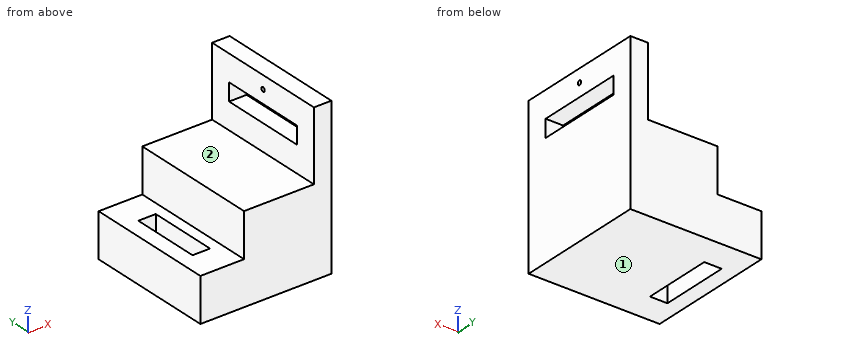
```python
from build123d import *

# Parameters (mm, degrees)
F1_DEPTH = 150
F2_W     = 100
F2_H     = 20
F3_DEPTH = 20.001
F4_R     = 2.5
F5_DEPTH = 20.001
F6_W     = 20
F6_H     = 80
F7_DEPTH = 25.4
F8_W     = 20
F8_H     = 80
F9_DEPTH = 75.401


with BuildPart() as f1:
    # F0 (on Front) → F1 (new body)
    with BuildSketch(Plane.XZ):
        Polygon((75, -90), (75, 90), (55, 90), (55, 10), (-25, 10), (-25, -40), (-75, -40), (-75, -90), align=None)
    extrude(amount=F1_DEPTH)

    # F2 (on face) → F3 (cut, through all)
    with BuildSketch(Plane(origin=(55, 0, 0), x_dir=(0, -1, 0), z_dir=(-1, 0, 0))):
        with Locations((75, 50)):
            Rectangle(F2_W, F2_H)
    extrude(amount=-F3_DEPTH, mode=Mode.SUBTRACT)

    # F4 (on face) → F5 (cut, through all)
    with BuildSketch(Plane(origin=(55, 0, 0), x_dir=(0, -1, 0), z_dir=(-1, 0, 0))):
        with Locations((75, 75)):
            Circle(F4_R)
    extrude(amount=-F5_DEPTH, mode=Mode.SUBTRACT)

    # F6 (on face) → F7 (join)
    with BuildSketch(Plane.XY.offset(-40)):
        with Locations((-47.3200663872, -75.7392449304)):
            Rectangle(F6_W, F6_H)
    extrude(amount=F7_DEPTH)

    # F8 (on face) → F9 (cut, through all)
    with BuildSketch(Plane.XY.offset(-14.6)):
        with Locations((-47.3200663872, -75.7392449304)):
            Rectangle(F8_W, F8_H)
    extrude(amount=-F9_DEPTH, mode=Mode.SUBTRACT)


solid = f1.part
```
For this review, take the finished solid that the model builds, in its own axes (mm). Face numbers are marked on the shaded views. A direction names the side the tool comes from. Coordinates: 2 decimals unless noted, no trailing zeros. Loops run counter-clockwise (first coordinate to the right, second up) from the corner with the lowest first, then second, coordinate; pieces in that order, holes last. Notation, with made-up numbers: (65, -24.5) - (94, -24.5) arc R17 cw to (94, -5.5) - close; hole circle Ø5 at (-31.75, 47.25). An arc over 180 degrees is marked (long way). Use one line per item in the form item = value. Start each with the question number.
1) Take a section at C-C (y = -104). State the section outline as (x, z) points.
2) Take a section at D-D (y = -75). State the section outline as (x, z) points.
3) Take a section at B-B (z = 75). State the section outline as (x, y) points.
4) For pin 1 (8 mm diameter, centred on x = 8, y = -55, fed in from +Z), flat-tipped, find the tip position at first contact; note if it passes through.
5) For the marked faces 1 and 2, list the 3-axis set-ups (+Z, -Z, +X, -X, +Y, -Y) from which the entire face can be reached by the end or side of a thin tool; tool diameter is ignored.
6) Take a section at A-A (x = -46). State the section outline as (y, z) points.
7) To check wall thickness, follow probe 1 along Z at (x, y) = (64, -75); probe 2 along X at (y, z) = (-80, 27); probe 3 along X at (y, z) = (-47, -49). State the ranges of each line that lie inside material, in increasing order. Write a range as from..to.
From the geometry:
q1.outline = (-75, -90) - (-57.32, -90) - (-57.32, -40) - (-75, -40) - close; (-37.32, -90) - (75, -90) - (75, 40) - (55, 40) - (55, 10) - (-25, 10) - (-25, -40) - (-37.32, -40) - close; (55, 60) - (75, 60) - (75, 90) - (55, 90) - close
q2.outline = (-75, -90) - (-57.32, -90) - (-57.32, -40) - (-75, -40) - close; (-37.32, -90) - (75, -90) - (75, 40) - (55, 40) - (55, 10) - (-25, 10) - (-25, -40) - (-37.32, -40) - close; (55, 60) - (75, 60) - (75, 72.5) - (55, 72.5) - close; (55, 77.5) - (75, 77.5) - (75, 90) - (55, 90) - close
q3.outline = (55, -150) - (75, -150) - (75, -77.5) - (55, -77.5) - close; (55, -72.5) - (75, -72.5) - (75, 0) - (55, 0) - close
q4.pin_1 = 10
q5.face_1 = -Z, +X, -X, +Y, -Y
q5.face_2 = +Z, -X, +Y, -Y
q6.outline = (-150, -90) - (-115.74, -90) - (-115.74, -40) - (-150, -40) - close; (-35.74, -90) - (0, -90) - (0, -40) - (-35.74, -40) - close
q7.probe_1 = -90..40, 60..72.5, 77.5..90
q7.probe_2 = 55..75
q7.probe_3 = -75..-57.32, -37.32..75
